Check sheet for the drawn part. Datum: minimum x, y, z corner. Units: mm. Give positions to 0.01 mm unless a question says otherwise; leave off trailing zeros. Order: outer loops, then holes, each group sorted by start corner. A loop starts at its lowest first (then second) coordinate and runs counter-clockwise, first axis right, second up. Notation, with made-up numbers: M -4,-11.75 L 28,-11.75 A7 cw 28,-0.75 Z; hole C 22.25,-25 d5. An arc over 180 degrees is marked long. Answer as CSV lines item,"result". Start each with the question number.
Q1. Go/stop test with flat-tipped pins: pin 1 (6 mm diameter, centred on x = 12, z = 17.5, fed in from -Y); pin 2 (5.5 mm diameter, centred on x = 9.5, y = 11, fed in from +Z). Record where each tip stops, or that it passes through.
Q2. Thickness scan on line 1 (X direction, y = 10, z = 14); line 2 (Z direction, x = 5.5, y = 37); line 3 (Z direction, x = 2.75, y = 16.5). Record the ranges inside material, lowest first.
Q3. Section check B-B, the plane y = 37.5. Record the boundary of the cut face in (x, z).
Q4. Section check A-A, the plane x = 7. Record the boundary of the cut face in (y, z).
Q5. Section check D-D, the plane z = 22. Record the boundary of the cut face in (x, y), then the cut area to 3 significant figures.
Q6. Section check C-C, the plane z = 6. Record the boundary of the cut face in (x, y).
Q7. Mould release check, pull along X, two halves, no side actions. Record for the marked faces 1, 2, 3 and 4: +X half, -X half, draft (parallel to the pull), parting line (faces both ways), or undercut.
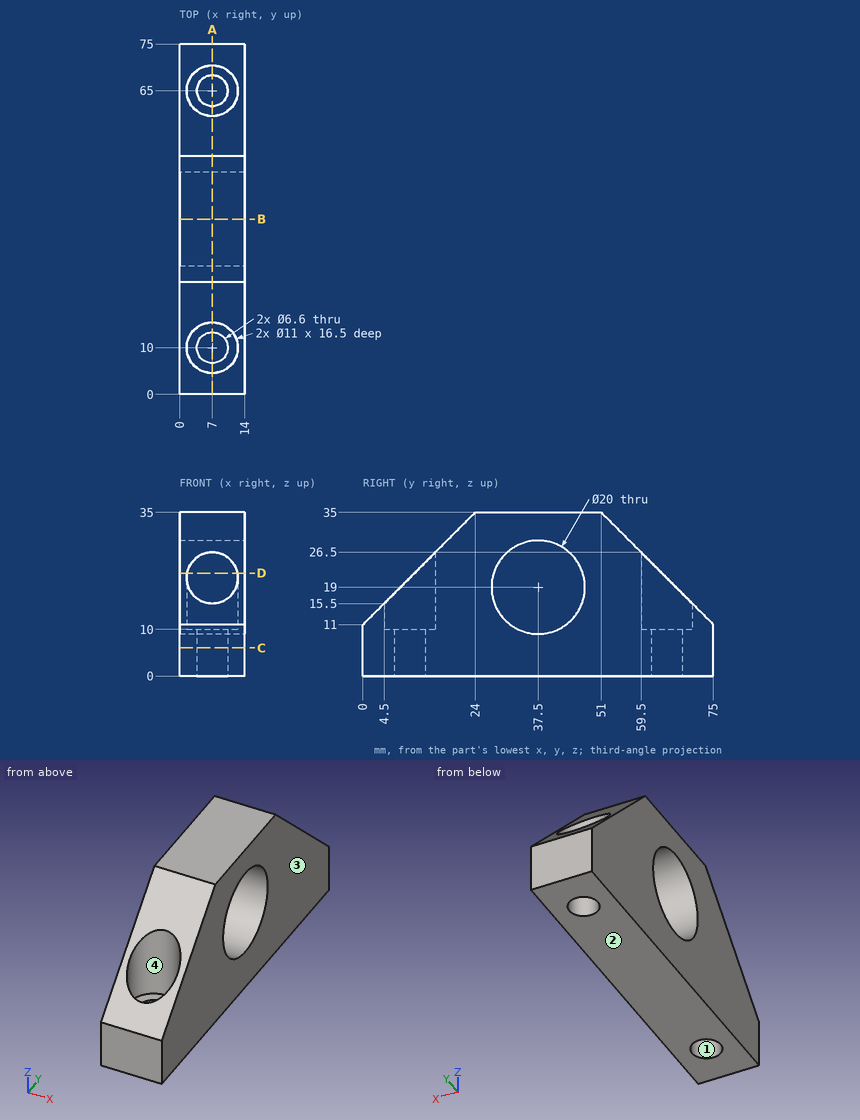
Answer block:
1,pin 1,"stops at y = 3.5"
1,pin 2,"stops at z = 10"
2,line 1,"x = 0 to 1.5, 12.5 to 14"
2,line 2,"z = 0 to 9.01, 28.99 to 35"
2,line 3,"z = 0 to 27.5"
3,outline,"M 0,0 L 14,0 L 14,9 L 0,9 Z; M 0,29 L 14,29 L 14,35 L 0,35 Z"
4,outline,"M 0,0 L 6.7,0 L 6.7,10 L 4.5,10 L 4.5,15.5 L 0,11 Z; M 13.3,0 L 61.7,0 L 61.7,10 L 59.5,10 L 59.5,26.5 L 51,35 L 24,35 L 15.5,26.5 L 15.5,10 L 13.3,10 Z; M 68.3,0 L 75,0 L 75,11 L 70.5,15.5 L 70.5,10 L 68.3,10 Z; hole C 37.5,19 d20"
5,outline,"M 0,11 L 1.59,11 A5.5 cw 12.41,11 L 14,11 L 14,27.96 L 0,27.96 Z; M 0,47.04 L 14,47.04 L 14,64 L 12.41,64 A5.5 cw 1.59,64 L 0,64 Z"
5,area,"402 mm2"
6,outline,"M 0,0 L 14,0 L 14,75 L 0,75 Z; hole C 7,10 d6.6; hole C 7,65 d6.6"
7,face 1,"undercut"
7,face 2,"draft"
7,face 3,"+X half"
7,face 4,"undercut"
